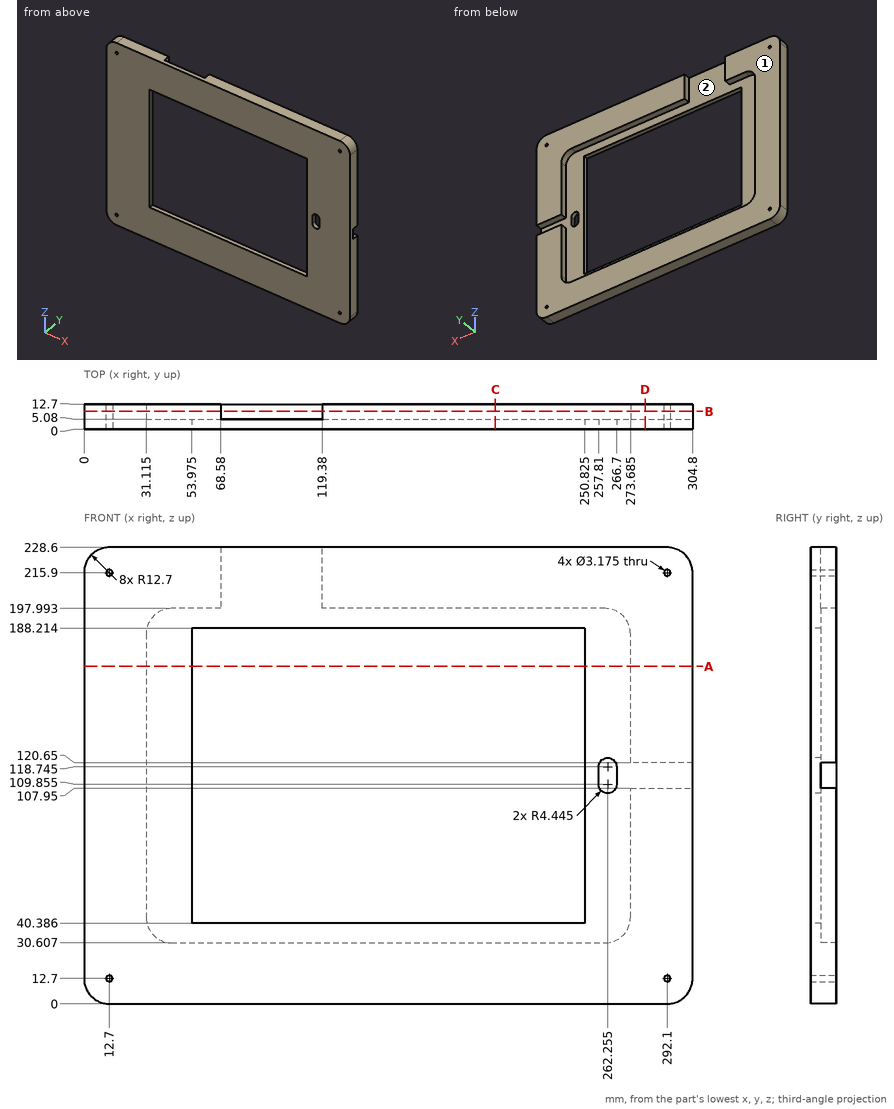
Geometry check sheet. Reference: drawing and pictorial views, mm from the part's lowest x, y, z. Round coordinates to 2 decimals unless told otherwise and drop trailing zeros. Write each loop counter-clockwise with the first axis right and the second up, starting at its lowest first coordinate (ties: lowest second). Pieces come first, ordered by that corner, then holes.
1. Section check B-B on y = 9. State how many separate pieces and enclosed holes the cut face has, plus the area to 3 significant figures.
2. Section check D-D on x = 281. Enter the section's corners in (y, z), plus the area to 3 significant figures.
3. Gauge pin test, flat ends, axial feed: P1, Ø8, axis at x = 140.5, z = 33.5, coming from the +Y side; P2, Ø2.5, axis at y = 7.5, z = 111.5, coming from the +X side (3 decimals); P3, Ø3, axis at x = 292.1, z = 215.9, coming from the +Y side. Record the tip position at first contact, or that the pin passes through.
4. Scan lines: L1, parallel to X at y = 6.25, z = 215.9; L2, parallel to X at y = 10.25, z = 136.5 (3 decimals); L3, parallel to Z at x = 161, y = 4. Record each from-to range of solid material in increasing order.
5. Section check A-A on z = 169. Enter the section's corners in (x, y) (3 decimals), plus the area to 3 significant figures.
6. Draft check along Z on the marked faces 1 and 2. Enter one of: +Z half, -Z half, draft (parallel to the pull), parting line (faces both ways), or undercut.
7. Section check C-C on x = 206. Enter the section's corners in (y, z), plus the area to 3 significant figures.
Answer:
1. separate pieces: 2
1. enclosed holes: 4
1. area: 27,100 mm2
2. outline: (0, 0) - (12.7, 0) - (12.7, 107.95) - (5.08, 107.95) - (5.08, 120.65) - (12.7, 120.65) - (12.7, 228.6) - (0, 228.6) - close
2. area: 2,810 mm2
3. P1: stops at y = 12.7
3. P2: stops at x = 31.115
3. P3: passes through
4. L1: x = 0 to 11.11, 14.29 to 68.58, 119.38 to 290.51, 293.69 to 304.8
4. L2: x = 0 to 31.115, 273.685 to 304.8
4. L3: z = 0 to 40.39, 188.21 to 228.6
5. outline: (0, 0) - (53.975, 0) - (53.975, 5.08) - (31.115, 5.08) - (31.115, 12.7) - (0, 12.7) - close; (250.825, 0) - (304.8, 0) - (304.8, 12.7) - (273.685, 12.7) - (273.685, 5.08) - (250.825, 5.08) - close
5. area: 1,020 mm2
6. face 1: draft
6. face 2: undercut
7. outline: (0, 0) - (12.7, 0) - (12.7, 30.61) - (5.08, 30.61) - (5.08, 40.39) - (0, 40.39) - close; (0, 188.21) - (5.08, 188.21) - (5.08, 197.99) - (12.7, 197.99) - (12.7, 228.6) - (0, 228.6) - close
7. area: 877 mm2
